For this review, use the dimensioned drawing (mm, ordinates from the lowest corner) and the shaded views. A direction names the side the tool comes from. Give positions to 0.01 mm unless a question says otherwise; leave off trailing zeros. Write each loop counter-clockwise with the first axis right and the second up, starting at its lowest first coordinate (ties: lowest second). Pieces come first, ordered by that corner, then holes.
1) We need section C-C on x = 51. Give the boundary of the cut face in (y, z), and give its area (3 significant figures).
2) We need section B-B on y = 63.5. Give the boundary of the cut face in (x, z), and give its area (3 significant figures).
3) Wall thickness on line 1 along X through (y, z) = (22.5, 15.75); line 2 along Y through (x, z) = (34, 3.5); line 3 along Z through (x, y) = (53, 46): over which ranges is each line inside the solid? List them lowest first.
4) Machinability: for the marked faces 1 and 2, which of the approach directions +Z, -Z, +X, -X, +Y, -Y give a long, thin tool a straight path to every point of the face, cutting with its end or side? Answer none if there is none.
5) We need section A-A on z = 16. Give the boundary of the cut face in (x, y).
6) For P1, Ø5, axis at x = 27, z = 11.5, coming from the -Y side; P2, Ø10, axis at x = 69, y = 19, coming from the +Z side, all flat-tipped, find the tip position at first contact; note any pin that passes through.
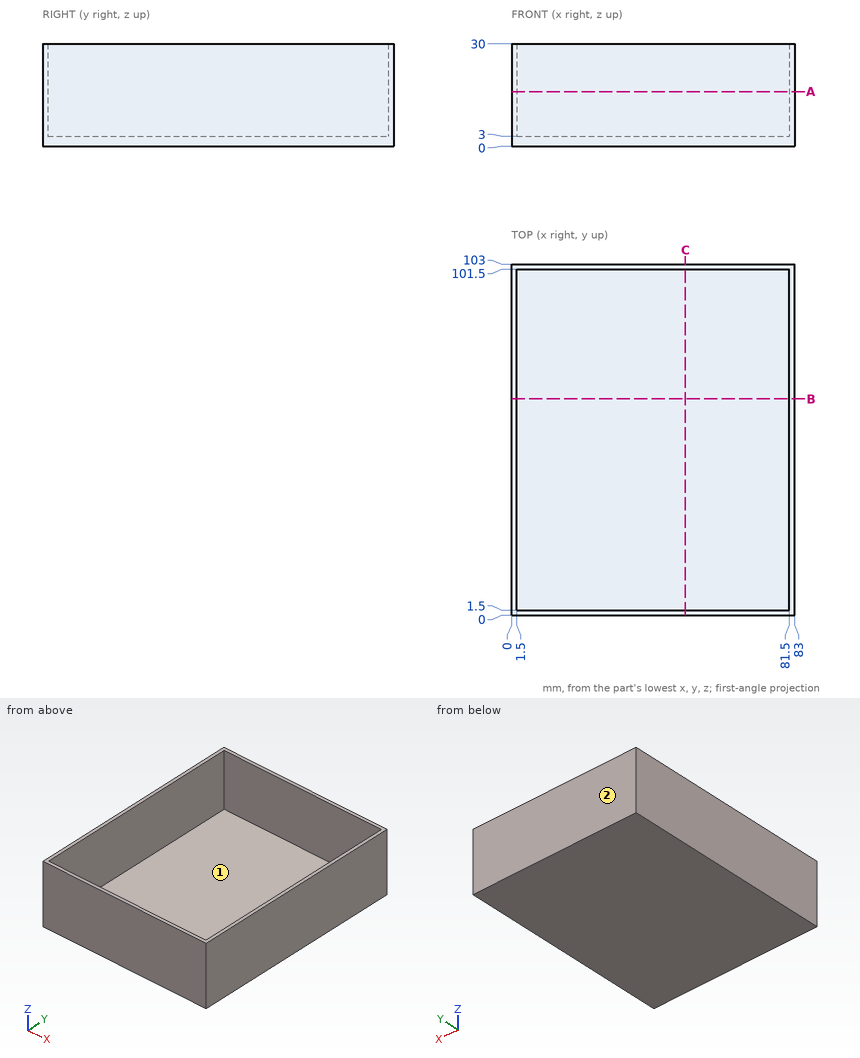
Results list:
1. outline: (0, 0) - (103, 0) - (103, 30) - (101.5, 30) - (101.5, 3) - (1.5, 3) - (1.5, 30) - (0, 30) - close
1. area: 390 mm2
2. outline: (0, 0) - (83, 0) - (83, 30) - (81.5, 30) - (81.5, 3) - (1.5, 3) - (1.5, 30) - (0, 30) - close
2. area: 330 mm2
3. line 1: x = 0 to 1.5, 81.5 to 83
3. line 2: y = 0 to 1.5, 101.5 to 103
3. line 3: z = 0 to 3
4. face 1: +Z
4. face 2: +Z, -Z, +X, -X, +Y
5. outline: (0, 0) - (83, 0) - (83, 103) - (0, 103) - close; hole (1.5, 1.5) - (81.5, 1.5) - (81.5, 101.5) - (1.5, 101.5) - close
6. P1: stops at y = 0
6. P2: stops at z = 3
